The listing builds one solid part. Answer for the finished solid, in the listing's coordinates (mm). Face numbers are marked on the shaded views. A direction names the side the tool comes from. Coordinates: 2 decimals unless noted, no trailing zeros. Order: outer loops, then holes, each group sorted by start corner. A loop starts at its lowest first (then second) coordinate and runs counter-clockwise, first axis right, second up.
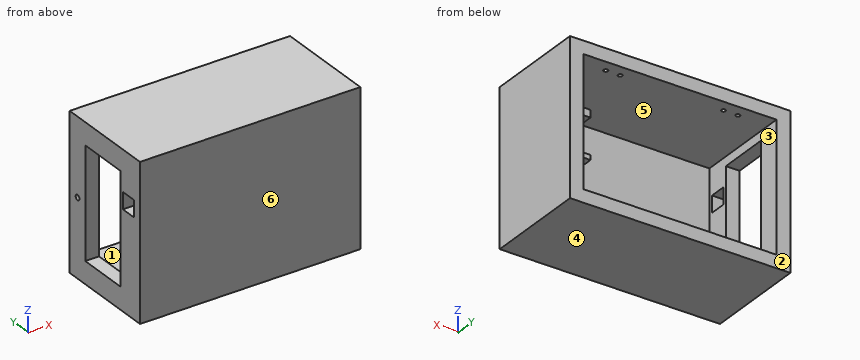
```python
from build123d import *

# Parameters (mm, degrees)
SKETCH2_W                = 152.4
SKETCH2_H                = 106.68
BOSS_EXTRUDE1_DEPTH      = 71.12
SKETCH3_W                = 133.35
SKETCH3_H                = 88.9
CUT_EXTRUDE1_DEPTH       = 67.945
SKETCH8_W                = 5.08
SKETCH8_H                = 24.765
SKETCH8_W_2              = 3.302
SKETCH8_H_2              = 49.53
BOSS_EXTRUDE2_DEPTH      = 17.272
SKETCH12_W               = 76.2
SKETCH12_H               = 35.56
CUT_EXTRUDE3_DEPTH       = 9.525
CUT_EXTRUDE12_DEPTH      = 93.820000066
CUT_EXTRUDE12_DEPTH_BACK = 4.45999997
SKETCH35_R               = 1.4986
SKETCH36_R               = 1.905
CUT_EXTRUDE13_DEPTH      = 2.54
SKETCH37_W               = 11.43
SKETCH37_H               = 11.43
CUT_EXTRUDE14_DEPTH      = 9.525


with BuildPart() as part:
    # Sketch2 → Boss-Extrude1 (new body)
    with BuildSketch(Plane(origin=(0, 0, 0), x_dir=(1, 0, 0), z_dir=(0, 1, 0))):
        with Locations((76.2, -53.34)):
            Rectangle(SKETCH2_W, SKETCH2_H)
    extrude(amount=BOSS_EXTRUDE1_DEPTH)

    # Sketch3 → Cut-Extrude1 (cut)
    with BuildSketch(Plane(origin=(0, 71.12, 0), x_dir=(1, 0, 0), z_dir=(0, 1, 0))):
        with Locations((76.2, -53.34)):
            Rectangle(SKETCH3_W, SKETCH3_H)
    extrude(amount=-CUT_EXTRUDE1_DEPTH, mode=Mode.SUBTRACT)

    # Sketch8 → Boss-Extrude2 (add)
    with BuildSketch(Plane.ZY.offset(-142.875)):
        with Locations((72.898, 40.3225)):
            Rectangle(SKETCH8_W, SKETCH8_H)
        with Locations((72.898, 15.5575)):
            Rectangle(SKETCH8_W, SKETCH8_H)
        with Locations((44.069, 27.94)):
            Rectangle(SKETCH8_W_2, SKETCH8_H_2)
    extrude(amount=BOSS_EXTRUDE2_DEPTH)

    # Sketch12 → Cut-Extrude3 (cut)
    with BuildSketch(Plane.ZY):
        with Locations((53.34, 37.592)):
            Rectangle(SKETCH12_W, SKETCH12_H)
    extrude(amount=-CUT_EXTRUDE3_DEPTH, mode=Mode.SUBTRACT)

    # Sketch35 → Cut-Extrude12 (cut, two sides: drawn at the far end of the back side and taken through both)
    with BuildSketch(Plane.XY.offset(8.89).offset(-CUT_EXTRUDE12_DEPTH_BACK)):
        with Locations(Location((30.48, 62.738, 0), (0, 0, 180))):
            Circle(SKETCH35_R)
        with Locations(Location((40.4876, 62.738, 0), (0, 0, 180))):
            Circle(SKETCH35_R)
        with Locations(Location((111.9124, 62.738, 0), (0, 0, 180))):
            Circle(SKETCH35_R)
        with Locations(Location((121.92, 62.738, 0), (0, 0, 180))):
            Circle(SKETCH35_R)
    extrude(amount=CUT_EXTRUDE12_DEPTH + CUT_EXTRUDE12_DEPTH_BACK, mode=Mode.SUBTRACT)

    # Sketch36 → Cut-Extrude13 (cut)
    with BuildSketch(Plane.ZY):
        with Locations((53.34, 63.221423834)):
            Circle(SKETCH36_R)
    extrude(amount=-CUT_EXTRUDE13_DEPTH, mode=Mode.SUBTRACT)

    # Sketch37 → Cut-Extrude14 (cut)
    with BuildSketch(Plane.ZY):
        with Locations((73.025, 11.557)):
            Rectangle(SKETCH37_W, SKETCH37_H)
    extrude(amount=-CUT_EXTRUDE14_DEPTH, mode=Mode.SUBTRACT)


solid = part.part
```
1) A cutting plane is placed at B-B, the plane y = 27. Write down the section's boundary in (x, z) (3 decimals).
2) A cutting plane is placed at D-D, the plane z = 96. Write down the section's boundary in (x, y) (3 decimals), plus the area to 3 significant figures.
3) For the marked faces 5 and 6, determine the directions among +Z, -Z, +X, -X, +Y, -Y from which every point of the face is accessible in a straight line to the end or side of a thin tool.
4) A cutting plane is placed at A-A, the plane z = 64. Write down the section's boundary in (x, y) (3 decimals).
5) Straight lines are drawn through the part: probe 1 along Y at (x, z) = (1.7, 53.34); probe 2 along Z at (x, y) = (126.5, 16); probe 3 along Y at (x, z) = (30.48, 7.4). For each, find the intervals that lie inside material, in ascending order.
6) A cutting plane is placed at C-C, the plane x = 98. Write down the section's boundary in (y, z) (3 decimals), plus the area to 3 significant figures.
7) The mould has two halves that part along Z. Classify the marked faces 1, 2, 3 and 4: released by +Z, released by -Z, zero draft, split by the parting line, or undercut.
8) Each of these flat-tipped pins is pushed along its axis until it touches: P1, Ø5, axis at y = 42, z = 76.5, coming from the -X side; P2, Ø1, axis at x = 60.5, z = 19.5, coming from the +Y side (3 decimals); P3, Ø1, axis at x = 136.5, z = 44.5, coming from the +Y side (3 decimals); P4, Ø3, axis at x = 52.5, y = 27.5, coming from the -Z side. Where does it stop, or does it pass through?
Working result:
1. outline: (0, 0) - (152.4, 0) - (152.4, 106.68) - (0, 106.68) - (0, 91.44) - (9.525, 91.44) - (9.525, 97.79) - (142.875, 97.79) - (142.875, 75.438) - (125.603, 75.438) - (125.603, 70.358) - (142.875, 70.358) - (142.875, 45.72) - (125.603, 45.72) - (125.603, 42.418) - (142.875, 42.418) - (142.875, 8.89) - (9.525, 8.89) - (9.525, 15.24) - (0, 15.24) - close
2. outline: (0, 0) - (152.4, 0) - (152.4, 71.12) - (142.875, 71.12) - (142.875, 3.175) - (9.525, 3.175) - (9.525, 71.12) - (0, 71.12) - close
2. area: 1,780 mm2
3. face 5: +Y
3. face 6: +Z, -Z, +X, -X, -Y
4. outline: (0, 0) - (152.4, 0) - (152.4, 71.12) - (142.875, 71.12) - (142.875, 3.175) - (9.525, 3.175) - (9.525, 19.812) - (0, 19.812) - close; (0, 55.372) - (9.525, 55.372) - (9.525, 71.12) - (0, 71.12) - close
5. probe 1: y = 0 to 19.81, 55.37 to 61.32, 65.13 to 71.12
5. probe 2: z = 0 to 8.89, 42.42 to 45.72, 70.36 to 75.44, 97.79 to 106.68
5. probe 3: y = 0 to 61.24, 64.24 to 71.12
6. outline: (0, 0) - (71.12, 0) - (71.12, 8.89) - (3.175, 8.89) - (3.175, 97.79) - (71.12, 97.79) - (71.12, 106.68) - (0, 106.68) - close
6. area: 1,550 mm2
7. face 1: undercut
7. face 2: zero draft
7. face 3: undercut
7. face 4: released by -Z
8. P1: stops at x = 125.6
8. P2: stops at y = 3.175
8. P3: stops at y = 52.705
8. P4: stops at z = 0
